```python
from build123d import *

# Parameters (mm, degrees)
F0_W     = 24.7
F0_H     = 16.1
F1_DEPTH = 1.5
F0_W_2   = 51.9
F0_H_2   = 1.5
F2_DEPTH = 21.8
F0_W_3   = 61.7
F3_DEPTH = 21.8
F4_R     = 2
F6_D     = 5
F6_DEPTH = 100
F7_D     = 3
F7_DEPTH = 100
F8_D     = 3


with BuildPart() as f1:
    # F0 (on Front) → F1 (new body)
    with BuildSketch(Plane.XZ):
        Polygon((30.85, 11.05), (-30.85, 11.05), (-30.85, -4.95), (-21.05, -4.95), (-21.05, -11.05), (30.85, -11.05), align=None)
        with BuildLine():
            ThreePointArc((-20.95, 0), (-20.975212, -0.273861), (-21.05, -0.538516))
            ThreePointArc((-21.05, -0.538516), (-23.95, 0), (-21.05, 0.538516))
            ThreePointArc((-21.05, 0.538516), (-20.975212, 0.273861), (-20.95, 0))
        make_face(mode=Mode.SUBTRACT)
        with Locations((13.35, 0)):
            Rectangle(F0_W, F0_H, mode=Mode.SUBTRACT)
    extrude(amount=F1_DEPTH)

    # F0 (on Front) → F2 (join)
    with BuildSketch(Plane.XZ):
        with Locations((4.9, -11.8)):
            Rectangle(F0_W_2, F0_H_2)
    extrude(amount=F2_DEPTH)

    # F0 (on Front) → F3 (join)
    with BuildSketch(Plane.XZ):
        with Locations((0, 11.8)):
            Rectangle(F0_W_3, F0_H_2)
    extrude(amount=F3_DEPTH)

    # F4
    f4_edges = [f1.edges().sort_by_distance(p)[0] for p in [
        (0, 0, 12.55),
        (4.9, 0, -12.55),
    ]]
    fillet(f4_edges, radius=F4_R)

    # F6
    with Locations(Plane.XY.offset(12.55)):
        with Locations((-13.863446, -13.334782)):
            Hole(F6_D / 2, depth=F6_DEPTH)

    # F7
    with Locations(Plane.XY.offset(12.55)):
        with Locations((16.783738, -4.766752)):
            Hole(F7_D / 2, depth=F7_DEPTH)

    # F8 (through all)
    with Locations(Plane.XY.offset(12.55)):
        with Locations((-18.35013, -5.2)):
            Hole(F8_D / 2)


solid = f1.part
```
Geometry: final body of the model. Coordinates: model frame, mm. A direction names the side the tool comes from. Coordinates: 2 decimals unless noted, no trailing zeros. Order: outer loops, then holes, each group sorted by start corner. A loop starts at its lowest first (then second) coordinate and runs counter-clockwise, first axis right, second up. Notation, with made-up numbers: M 53.25,-32.5 L 92.25,-32.5 A30 ccw 92.25,-1.5 Z; hole C -3.5,-22.5 d9. An arc over 180 degrees is marked long. Answer in a Markdown table with one row per item. Add a question column.
Q1. Section query D-D on y = -12. Return the cut outline in (x, z).
Q2. Mould query, pull axis X, two halves, no side actions, for faces 4 (the cylindrical face through (-15.02, -15.55, -11.81)), 5 (the flat face through (5, -21.8, -12)), 6 (the flat face through (-30.85, -6, 12)). Classes: released by +X, released by -X, zero draft, split by the parting line, or undercut.
Q3. Reachability of faces 1 (the flat face through (-26, -1, -4.95)), 2 (the flat face through (0, -12, 11.05)), 3 (the flat face through (13, -1, -8.05)) from +Z, -Z, +X, -X, +Y, -Y: full face, straight path, thin tool, end or side. Return the list, or none.
Q4. Section query B-B on x = -22.45. Return the cut outline in (y, z).
Q5. Line query: L1, parallel to X at y = -1.05, z = 0; L2, parallel to Z at x = -5, y = -18. Output: solid intervals per line, ascending.
Q6. Contact query for flat-ended pins moving along their axis: P1, Ø6.5, axis at x = 10, z = -3, coming from the -Y side; P2, Ø0.8, axis at x = -24.5, y = -1, coming from the -Z side; P3, Ø1, axis at x = -23.5, z = -0.5, coming from the -Y side; P4, Ø0.8, axis at x = 16, y = -0.5, coming from the +Z side. Output: stop coordinate, or through.
Q7. Section query C-C on z = 2.75. Return the cut outline in (x, y), and give its area (3 significant figures).
Q8. Section query A-A on y = -8.5. Return the cut outline in (x, z).
Completed:
| question | item | result |
|---|---|---|
| 1 | outline | M -30.85,11.05 L -15.98,11.05 L -15.98,12.55 L -30.85,12.55 Z; M -21.05,-12.55 L -15.98,-12.55 L -15.98,-11.05 L -21.05,-11.05 Z; M -11.75,-12.55 L 30.85,-12.55 L 30.85,-11.05 L -11.75,-11.05 Z; M -11.75,11.05 L 30.85,11.05 L 30.85,12.55 L -11.75,12.55 Z |
| 2 | face 4 | undercut |
| 2 | face 5 | zero draft |
| 2 | face 6 | released by -X |
| 3 | face 1 | -Z, -X, +Y, -Y |
| 3 | face 2 | +X, -X, -Y |
| 3 | face 3 | +Y, -Y |
| 4 | outline | M -21.8,11.05 L -1.5,11.05 L -1.5,1.5 L 0,1.5 L 0,10.55 A2 ccw -2,12.55 L -21.8,12.55 Z; M -1.5,-4.95 L 0,-4.95 L 0,-1.5 L -1.5,-1.5 Z |
| 5 | L1 | x = -30.85 to -23.95, -20.95 to 1, 25.7 to 30.85 |
| 5 | L2 | z = -12.55 to -11.05, 11.05 to 12.55 |
| 6 | P1 | passes through |
| 6 | P2 | stops at z = -4.95 |
| 6 | P3 | stops at y = -1.5 |
| 6 | P4 | stops at z = 12.22 |
| 7 | outline | M -30.85,-1.5 L 1,-1.5 L 1,0 L -30.85,0 Z; M 25.7,-1.5 L 30.85,-1.5 L 30.85,0 L 25.7,0 Z |
| 7 | area | 55.5 mm2 |
| 8 | outline | M -30.85,11.05 L 30.85,11.05 L 30.85,12.55 L -30.85,12.55 Z; M -21.05,-12.55 L 30.85,-12.55 L 30.85,-11.05 L -21.05,-11.05 Z |
